from build123d import *

# Parameters (mm, degrees)
SKETCH1_W           = 150
SKETCH1_H           = 70
BOSS_EXTRUDE1_DEPTH = 10
SKETCH2_W           = 18
SKETCH2_H           = 70
BOSS_EXTRUDE2_DEPTH = 80
FILLET1_R           = 35
SKETCH3_R           = 6.5
CUT_EXTRUDE1_DEPTH  = 164.102034121
RIB1_REACH          = 134.904
SKETCH5_WALL_W      = 321.142477346
SKETCH5_WALL_H      = 40
SKETCH7_W           = 43.830511012
SKETCH7_H           = 10.028409091
CUT_EXTRUDE2_DEPTH  = 80
SCALE1_SCALE        = 0.31
CUT_EXTRUDE5_REACH  = 46.882
SKETCH11_W          = 1.005
SKETCH11_H          = 10.85
SKETCH11_H_2        = 13.95
BOSS_EXTRUDE3_DEPTH = 20


with BuildPart() as part:
    # Sketch1 → Boss-Extrude1 (new body)
    with BuildSketch(Plane(origin=(0, 0, 0), x_dir=(1, 0, 0), z_dir=(0, 1, 0))):
        with Locations((14.225473782, -5.028409091)):
            Rectangle(SKETCH1_W, SKETCH1_H)
    extrude(amount=BOSS_EXTRUDE1_DEPTH)

    # Sketch2 → Boss-Extrude2 (add)
    with BuildSketch(Plane(origin=(0, 10, 0), x_dir=(1, 0, 0), z_dir=(0, 1, 0))):
        with Locations((-31.774526218, -5.028409091)):
            Rectangle(SKETCH2_W, SKETCH2_H)
        with Locations((21.225473782, -5.028409091)):
            Rectangle(SKETCH2_W, SKETCH2_H)
    extrude(amount=BOSS_EXTRUDE2_DEPTH)

    # Fillet1
    fillet1_edges = [part.edges().sort_by_distance(p)[0] for p in [
        (21.225473782, 90, 40.028409091),
        (21.225473782, 90, -29.971590909),
        (-31.774526218, 90, -29.971590909),
        (-31.774526218, 90, 40.028409091),
    ]]
    fillet(fillet1_edges, radius=FILLET1_R - 0.0001)  # a hair under: the kernel refuses the full size

    # Sketch3 → Cut-Extrude1 (cut, through all)
    with BuildSketch(Plane.ZY.offset(40.774526218)):
        with Locations((5.212032143, 50)):
            Circle(SKETCH3_R)
    extrude(amount=-CUT_EXTRUDE1_DEPTH, mode=Mode.SUBTRACT)

    # Sketch5 wall → Rib1 (add, up to next)
    with BuildSketch(Plane(origin=(52.140729288, 25.194278726, 0), x_dir=(0.821802771323, -0.569772064116, 0), z_dir=(0.569772064116, 0.821802771323, 0)), mode=Mode.PRIVATE) as rib1_sk1:
        Rectangle(SKETCH5_WALL_W, SKETCH5_WALL_H)
    rib1_tool1 = extrude(rib1_sk1.sketch, amount=-RIB1_REACH, mode=Mode.PRIVATE) - part.part
    add(rib1_tool1.solids().sort_by_distance((52.140729288, 25.194278726, 0))[0])

    # Sketch7 → Cut-Extrude2 (cut)
    with BuildSketch(Plane(origin=(0, 10, 0), x_dir=(1, 0, 0), z_dir=(0, 1, 0))):
        with Locations((52.140729288, 14.985795454)):
            Rectangle(SKETCH7_W, SKETCH7_H)
    extrude(amount=CUT_EXTRUDE2_DEPTH, mode=Mode.SUBTRACT)


with BuildPart() as part_1:
    # Scale1: scaled about (0, 0, 0)
    add(part.part.scale(SCALE1_SCALE))

    # Sketch11 → Cut-Extrude5 (cut, up to next)
    with BuildSketch(Plane(origin=(0, 0, -9.291193182), x_dir=(-1, 0, 0), z_dir=(0, 0, -1)), mode=Mode.PRIVATE) as cut_extrude5_sk1:
        Polygon((-9.369896872, 3.1), (-8.364896872, 3.1), (-8.364896872, 17.05), (-9.369896872, 17.05), (-9.369896872, 12.52045281), align=None)
    cut_extrude5_tool1 = extrude(cut_extrude5_sk1.sketch, amount=-CUT_EXTRUDE5_REACH, mode=Mode.PRIVATE) & part_1.part
    # Sketch11 → Cut-Extrude5 (cut, up to next)
    with BuildSketch(Plane(origin=(0, 0, -9.291193182), x_dir=(-1, 0, 0), z_dir=(0, 0, -1)), mode=Mode.PRIVATE) as cut_extrude5_sk2:
        with Locations((-8.867396872, 22.475)):
            Rectangle(SKETCH11_W, SKETCH11_H)
    cut_extrude5_tool2 = extrude(cut_extrude5_sk2.sketch, amount=-CUT_EXTRUDE5_REACH, mode=Mode.PRIVATE) & part_1.part
    # Sketch11 → Cut-Extrude5 (cut, up to next)
    with BuildSketch(Plane(origin=(0, 0, -9.291193182), x_dir=(-1, 0, 0), z_dir=(0, 0, -1)), mode=Mode.PRIVATE) as cut_extrude5_sk3:
        Polygon((-22.957355286, 3.1), (-9.369896872, 3.1), (-9.369896872, 12.52045281), align=None)
    cut_extrude5_tool3 = extrude(cut_extrude5_sk3.sketch, amount=-CUT_EXTRUDE5_REACH, mode=Mode.PRIVATE) & part_1.part
    # Sketch11 → Cut-Extrude5 (cut, up to next)
    with BuildSketch(Plane(origin=(0, 0, -9.291193182), x_dir=(-1, 0, 0), z_dir=(0, 0, -1)), mode=Mode.PRIVATE) as cut_extrude5_sk4:
        Polygon((-8.364896872, 0), (-8.364896872, 3.1), (-9.369896872, 3.1), (-22.957355286, 3.1), (-27.659896872, 3.1), (-27.659896872, 0), align=None)
    cut_extrude5_tool4 = extrude(cut_extrude5_sk4.sketch, amount=-CUT_EXTRUDE5_REACH, mode=Mode.PRIVATE) & part_1.part
    # Sketch11 → Cut-Extrude5 (cut, up to next)
    with BuildSketch(Plane(origin=(0, 0, -9.291193182), x_dir=(-1, 0, 0), z_dir=(0, 0, -1)), mode=Mode.PRIVATE) as cut_extrude5_sk5:
        with Locations((12.137603128, 10.075)):
            Rectangle(SKETCH11_W, SKETCH11_H_2)
    cut_extrude5_tool5 = extrude(cut_extrude5_sk5.sketch, amount=-CUT_EXTRUDE5_REACH, mode=Mode.PRIVATE) & part_1.part
    # Sketch11 → Cut-Extrude5 (cut, up to next)
    with BuildSketch(Plane(origin=(0, 0, -9.291193182), x_dir=(-1, 0, 0), z_dir=(0, 0, -1)), mode=Mode.PRIVATE) as cut_extrude5_sk6:
        with Locations((12.137603128, 22.475)):
            Rectangle(SKETCH11_W, SKETCH11_H)
    cut_extrude5_tool6 = extrude(cut_extrude5_sk6.sketch, amount=-CUT_EXTRUDE5_REACH, mode=Mode.PRIVATE) & part_1.part
    # Sketch11 → Cut-Extrude5 (cut, up to next)
    with BuildSketch(Plane(origin=(0, 0, -9.291193182), x_dir=(-1, 0, 0), z_dir=(0, 0, -1)), mode=Mode.PRIVATE) as cut_extrude5_sk7:
        Polygon((12.640103128, 3.1), (11.635103128, 3.1), (11.635103128, 0), (18.840103128, 0), (18.840103128, 3.1), align=None)
    cut_extrude5_tool7 = extrude(cut_extrude5_sk7.sketch, amount=-CUT_EXTRUDE5_REACH, mode=Mode.PRIVATE) & part_1.part
    add(cut_extrude5_tool1.solids().sort_by_distance((8.867397, 10.075, -9.291193))[0], mode=Mode.SUBTRACT)
    add(cut_extrude5_tool2.solids().sort_by_distance((8.867397, 22.475, -9.291193))[0], mode=Mode.SUBTRACT)
    add(cut_extrude5_tool3.solids().sort_by_distance((13.89905, 6.240151, -9.291193))[0], mode=Mode.SUBTRACT)
    add(cut_extrude5_tool4.solids().sort_by_distance((18.012397, 1.55, -9.291193))[0], mode=Mode.SUBTRACT)
    add(cut_extrude5_tool5.solids().sort_by_distance((-12.137603, 10.075, -9.291193))[0], mode=Mode.SUBTRACT)
    add(cut_extrude5_tool6.solids().sort_by_distance((-12.137603, 22.475, -9.291193))[0], mode=Mode.SUBTRACT)
    add(cut_extrude5_tool7.solids().sort_by_distance((-15.237603, 1.55, -9.291193))[0], mode=Mode.SUBTRACT)

    # Sketch13 → Boss-Extrude3 (add)
    with BuildSketch(Plane(origin=(8.364896872, 0, 0), x_dir=(0, 0, -1), z_dir=(1, 0, 0))):
        Polygon((1.566193182, -1.455), (1.566193182, 0), (-4.683806818, 0), (-4.683806818, -1.455), (-4.683806818, -1.8), (-4.683806818, -2.3), (-7.058806818, -2.3), (-7.058806818, -3.439339828), (-4.398146646, -6.1), (-1.768806818, -6.1), (-1.558806818, -6.31), (-1.348806818, -6.1), (1.28053301, -6.1), (3.941193182, -3.439339828), (3.941193182, -2.3), (1.566193182, -2.3), (1.566193182, -1.8), align=None)
    extrude(amount=-BOSS_EXTRUDE3_DEPTH)


solid = part_1.part
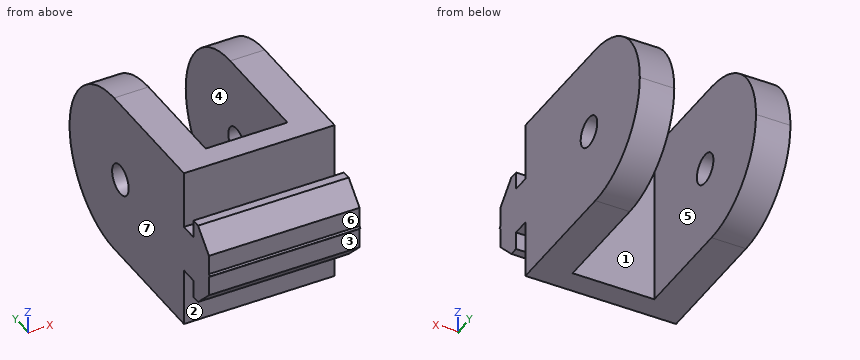
Can you work these out from the model? Positions are in its coordinate system, mm. Face numbers are marked on the shaded views. A direction names the side the tool comes from. Round coordinates to 2 decimals unless told otherwise and drop trailing zeros. Loops run counter-clockwise (first coordinate to the right, second up) from the corner with the lowest first, then second, coordinate; pieces in that order, holes last. Notation, with made-up numbers: (35, -30) - (52, -30) arc R10 cw to (52, -21) - close; hole circle Ø4 at (-15, 16.5). An arc over 180 degrees is marked (long way). Answer in a Markdown table with one row per item. Add a question column.
Q1. I want a section at C-C on z = -2.75. List the corners of the cut face in (x, y) for me, and give its area (3 significant figures).
Q2. We'd pull the mould along X, two halves only. Please class the marked faces 4, 5, 6 and 7: pulls with the +X half, pulls with the -X half, needs draft (parallel to the pull), parting line crosses it, or undercut.
Q3. For pin 1 Ø2.5 at (x, z) = (-1.5, 10) entering from -Y; pin 2 Ø0.6 at (x, y) = (-1, -3) entering from -Z; pin 3 Ø5.5 at (x, z) = (-4, -1) entering from +Y; pin 4 Ø1.2 at (x, y) = (-2.5, -0.5) entering from +Z, each with a flat end and sliding along its axis, tell me the tip position at first contact or that it passes through.
Q4. I want a section at B-B on y = 15.5. List the corners of the cut face in (x, z) for me, and give its area (3 significant figures).
Q5. Which directions (+Z, -Z, +X, -X, +Y, -Y) give clear straight access to the entire face, cutting with the end or side of a thin tool? Please do the marked faces 1, 2 and 3.
Q6. I need wall thicknesses on L1, parallel to X at y = 7, z = 6.5; L2, parallel to Y at x = 2.25, z = 8.5; L3, parallel to Y at x = -3.25, z = 0. Which ranges of each line are inside material? Lowest first, please.
Q7. I want a section at A-A on y = 5.5. List the corners of the cut face in (x, z) for me.
A:
| question | item | result |
|---|---|---|
| 1 | outline | (-11.64, -4.63) - (8.36, -4.63) - (8.36, -2.3) - (-11.64, -2.3) - close; (-11.64, 0) - (8.36, 0) - (8.36, 27.01) - (3.79, 27.01) - (3.79, 3.1) - (-7.06, 3.1) - (-7.06, 27.01) - (-11.64, 27.01) - close |
| 1 | area | 327 mm^2 |
| 2 | face 4 | undercut |
| 2 | face 5 | undercut |
| 2 | face 6 | needs draft |
| 2 | face 7 | pulls with the -X half |
| 3 | pin 1 | y = 0 |
| 3 | pin 2 | z = -3.94 |
| 3 | pin 3 | y = 3.1 |
| 3 | pin 4 | z = 12.41 |
| 4 | outline | (-11.64, -9.29) - (-7.06, -9.29) - (-7.06, -0.4) - (-11.64, -0.4) - close; (-11.64, 3.63) - (-7.06, 3.63) - (-7.06, 12.41) - (-11.64, 12.41) - close; (3.79, -9.29) - (8.36, -9.29) - (8.36, -0.4) - (3.79, -0.4) - close; (3.79, 3.63) - (8.36, 3.63) - (8.36, 12.41) - (3.79, 12.41) - close |
| 4 | area | 162 mm^2 |
| 5 | face 1 | +Z, -Z, +Y |
| 5 | face 2 | -Z, +X, -X |
| 5 | face 3 | -Z, +X, -X, -Y |
| 6 | L1 | -11.64 to -7.06, 3.79 to 8.36 |
| 6 | L2 | 0 to 3.1 |
| 6 | L3 | -6.1 to 3.1 |
| 7 | outline | (-11.64, -9.29) - (-7.06, -9.29) - (-7.06, 12.41) - (-11.64, 12.41) - close; (3.79, -9.29) - (8.36, -9.29) - (8.36, 12.41) - (3.79, 12.41) - close |
